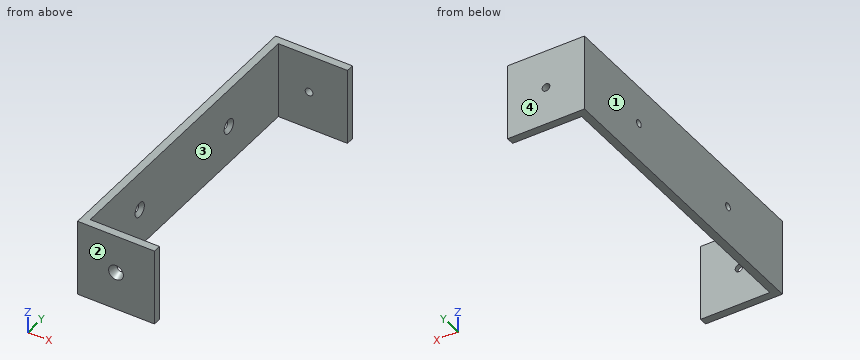
from build123d import *

# Parameters (mm, degrees)
SKETCH1_W                                           = 50
SKETCH1_H                                           = 50
BOSS_EXTRUDE1_DEPTH                                 = 200
SKETCH2_W                                           = 45
SKETCH2_H                                           = 190
CUT_EXTRUDE1_DEPTH                                  = 50
HOLE1_START                                         = 195
HOLE1_OUTLINE_R                                     = 2.5
HOLE1_DEPTH                                         = 5
SKETCH12_R                                          = 2.5
CUT_EXTRUDE2_DEPTH                                  = 5
CUT_EXTRUDE2_DRAFT                                  = 25
CSK_FOR_M4_COUNTERSUNK_FLAT_HEAD_SCREW1_D           = 4.8
CSK_FOR_M4_COUNTERSUNK_FLAT_HEAD_SCREW1_CSINK_D     = 9.4
CSK_FOR_M4_COUNTERSUNK_FLAT_HEAD_SCREW1_CSINK_ANGLE = 90


# Read off the part's stored shape, not the designer's step: Hole1
with BuildPart() as part:
    # Sketch1 → Boss-Extrude1 (new body)
    with BuildSketch(Plane(origin=(0, 0, 0), x_dir=(1, 0, 0), z_dir=(0, 1, 0))):
        with Locations((25, 25)):
            Rectangle(SKETCH1_W, SKETCH1_H)
    extrude(amount=BOSS_EXTRUDE1_DEPTH)

    # Sketch2 → Cut-Extrude1 (cut)
    with BuildSketch(Plane.XY):
        with Locations((27.5, 100)):
            Rectangle(SKETCH2_W, SKETCH2_H)
    extrude(amount=-CUT_EXTRUDE1_DEPTH, mode=Mode.SUBTRACT)

    # Hole1 outline → Hole1 (cut)
    with BuildSketch(Plane(origin=(0, 0, 0), x_dir=(1, 0, 0), z_dir=(0, 1, 0)).offset(HOLE1_START)):
        with Locations((25, 25)):
            Circle(HOLE1_OUTLINE_R)
    extrude(amount=HOLE1_DEPTH, mode=Mode.SUBTRACT)


with BuildPart() as cut_extrude2_tool:
    # Sketch12 → Cut-Extrude2 (with draft: the straight prism first)
    with BuildSketch(Plane(origin=(0, 5, 0), x_dir=(1, 0, 0), z_dir=(0, 1, 0))):
        with Locations(Location((25, 25, 0), (0, 0, 270))):
            Circle(SKETCH12_R)
    extrude(amount=-CUT_EXTRUDE2_DEPTH)
    # Cut-Extrude2: the draft: its side faces are tilted about the plane it starts from
    cut_extrude2_sides = [cut_extrude2_tool.faces().sort_by_distance(p)[0] for p in [
        (25, 2.5, -27.5),
    ]]
    draft(cut_extrude2_sides, Plane(origin=(0, 5, 0), x_dir=(1, 0, 0), z_dir=(0, 1, 0)), CUT_EXTRUDE2_DRAFT)


with BuildPart() as part_1:
    add(part.part)

    # Cut-Extrude2: cut by cut_extrude2_tool
    add(cut_extrude2_tool.part, mode=Mode.SUBTRACT)

    # CSK for M4 Countersunk Flat Head Screw1 (through all)
    with Locations(Plane(origin=(5, 0, 0), x_dir=(0, 0, -1), z_dir=(1, 0, 0))):
        with Locations((25, 145), (25, 55)):
            CounterSinkHole(CSK_FOR_M4_COUNTERSUNK_FLAT_HEAD_SCREW1_D / 2, CSK_FOR_M4_COUNTERSUNK_FLAT_HEAD_SCREW1_CSINK_D / 2, counter_sink_angle=CSK_FOR_M4_COUNTERSUNK_FLAT_HEAD_SCREW1_CSINK_ANGLE)


solid = part_1.part
Check sheet for the modelled part. Datum: model origin and axes. Units: mm. Face numbers are marked on the shaded views. Round coordinates to 2 decimals unless told otherwise and drop trailing zeros. Order: outer loops, then holes, each group sorted by start corner. A loop starts at its lowest first (then second) coordinate and runs counter-clockwise, first axis right, second up. Notation, with made-up numbers: M 57,89 L 101,89 A32 ccw 101,117 Z; hole C 37.25,73 d2. An arc over 180 degrees is marked long. One line per item, written item: value. Start each with the question number.
1. Gauge pin test, flat ends, axial feed: P1, Ø4, axis at y = 55, z = -25, coming from the +X side; P2, Ø1.5, axis at y = 38.5, z = -44.5, coming from the +X side. Record the tip position at first contact, or that the pin passes through.
2. Section check B-B on y = 145. Enter the section's corners in (x, z).
3. Section check D-D on x = 25. Enter the section's corners in (y, z).
4. Section check C-C on x = 33. Enter the section's corners in (y, z).
5. Section check A-A on z = -25. Enter the section's corners in (x, y).
6. Release check for a two-part mould opening along Y. For the marked faces 1, 2, 3 and 4 record: released by +Y, released by -Y, zero draft, split by the parting line, or undercut.
7. Scan lines: line 1 along Y through (x, z) = (8.5, -26); line 2 along Z through (x, y) = (25, 198.65); line 3 along Z through (x, y) = (2, 55). Record each from-to range of solid material in increasing order.
Results found:
1. P1: through
1. P2: x = 5
2. outline: M 0,-50 L 5,-50 L 5,-29.7 L 2.7,-27.4 L 0,-27.4 Z; M 0,-22.6 L 2.7,-22.6 L 5,-20.3 L 5,0 L 0,0 Z
3. outline: M 0,-50 L 5,-50 L 5,-27.5 L 0,-29.83 Z; M 0,-20.17 L 5,-22.5 L 5,0 L 0,0 Z; M 195,-50 L 200,-50 L 200,-27.5 L 195,-27.5 Z; M 195,-22.5 L 200,-22.5 L 200,0 L 195,0 Z
4. outline: M 0,-50 L 5,-50 L 5,0 L 0,0 Z; M 195,-50 L 200,-50 L 200,0 L 195,0 Z
5. outline: M 0,0 L 20.17,0 L 22.5,5 L 5,5 L 5,50.3 L 2.7,52.6 L 0,52.6 Z; M 0,57.4 L 2.7,57.4 L 5,59.7 L 5,140.3 L 2.7,142.6 L 0,142.6 Z; M 0,147.4 L 2.7,147.4 L 5,149.7 L 5,195 L 22.5,195 L 22.5,200 L 0,200 Z; M 27.5,5 L 29.83,0 L 50,0 L 50,5 Z; M 27.5,195 L 50,195 L 50,200 L 27.5,200 Z
6. face 1: zero draft
6. face 2: released by -Y
6. face 3: undercut
6. face 4: released by +Y
7. line 1: 0 to 5, 195 to 200
7. line 2: -50 to -27.5, -22.5 to 0
7. line 3: -50 to -27.4, -22.6 to 0
